from build123d import *

# Parameters (mm, degrees)
F1_DEPTH    = 2.54
F2_T1_DEPTH = 76.5641495789
F3_R        = 2.54
F4_DEPTH    = 2.54


# Not quite as in the source:
# - a fillet or chamfer that OpenCascade refuses, or shapes differently, is made with other operations: its cross-section is extruded or revolved along the edge and cut away or added


with BuildPart() as f1:
    # F0 (on Front) → F1 (new body)
    with BuildSketch(Plane.XZ):
        with BuildLine():
            Line((-63.5, 0), (0, 0))
            Line((0, 0), (-12.7, 19.05))
            Line((-12.7, 19.05), (-19.05, 19.05))
            Line((-19.05, 19.05), (-19.05, 13.97))
            ThreePointArc((-19.05, 13.97), (-22.225, 10.795), (-25.4, 13.97))
            Line((-25.4, 13.97), (-25.4, 19.05))
            Line((-25.4, 19.05), (-38.1, 19.05))
            Line((-38.1, 19.05), (-38.1, 13.97))
            ThreePointArc((-38.1, 13.97), (-41.275, 10.795), (-44.45, 13.97))
            Line((-44.45, 13.97), (-44.45, 19.05))
            Line((-44.45, 19.05), (-50.8, 19.05))
            Line((-50.8, 19.05), (-63.5, 0))
        make_face()
    extrude(amount=F1_DEPTH)

    # F2: chamfer of 2.54 on 2 edges, made by hand

    # F2_s2 → F2_t1 (cut)
    with BuildSketch(Plane.YZ.offset(-70.0320747894)):
        Polygon((0, 0), (-2.54, 2.54), (-2.54, 0), align=None)
        Polygon((-2.54, 0), (0, 2.54), (0, 0), align=None)
    extrude(amount=F2_T1_DEPTH, mode=Mode.SUBTRACT)

    # F3 (on face) → F4 (cut)
    with BuildSketch(Plane.XZ.offset(2.54)):
        with Locations((-12.7, 7.62)):
            Circle(F3_R)
        with Locations((-49.9533333333, 7.62)):
            Circle(F3_R)
    extrude(amount=-F4_DEPTH, mode=Mode.SUBTRACT)


solid = f1.part
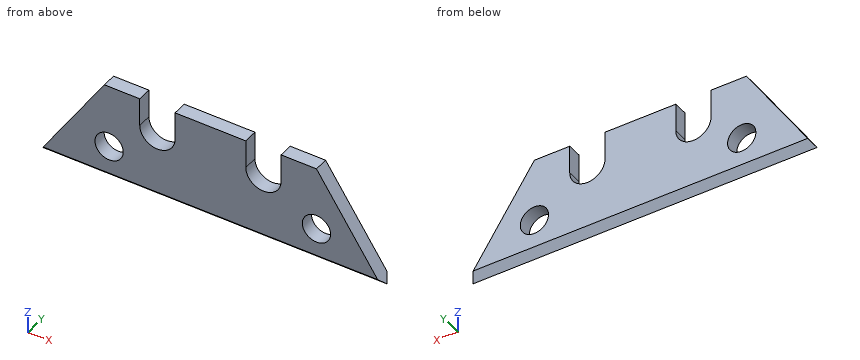
Model file for the job. Use its own axes, mm. Give positions to 0.01 mm unless a question says otherwise; leave off trailing zeros. Loops run counter-clockwise (first coordinate to the right, second up) from the corner with the lowest first, then second, coordinate; pieces in that order, holes last.
Item 1: Drop flat-ended pins along their axis: P1, Ø1.5, axis at y = -0.5, z = 11.5, coming from the -X side; P2, Ø0.8, axis at y = -2, z = 17.5, coming from the +X side; P3, Ø1.3, axis at y = -1.5, z = 16.5, coming from the -X side; P4, Ø4, axis at x = -49.95, z = 7.62, coming from the +Y side. Give the stop position or say it passes through.
Check values:
P1: stops at x = -56.33
P2: stops at x = -11.4
P3: stops at x = -52.93
P4: passes through
Item 2: Slice it at D-D (z = 12). Write the cut outline in (x, y).
Check values:
outline: (-55.5, -2.54) - (-43.76, -2.54) - (-43.76, 0) - (-55.5, 0) - close; (-38.79, -2.54) - (-24.71, -2.54) - (-24.71, 0) - (-38.79, 0) - close; (-19.74, -2.54) - (-8, -2.54) - (-8, 0) - (-19.74, 0) - close
Item 3: Slice it at C-C (x = -49). Write the cut outline in (y, z), plus the area to 3 significant figures.
Check values:
outline: (-2.54, 2.54) - (-1.27, 1.27) - (0, 2.54) - (0, 5.27) - (-2.54, 5.27) - close; (-2.54, 9.97) - (0, 9.97) - (0, 19.05) - (-2.54, 19.05) - close
area: 31.6 mm2
Item 4: Drill centre lines: line 1 along X through (y, z) = (-2.1, 16.5); line 2 along X through (y, z) = (-1.35, 14.25); line 3 along Z through (x, y) = (-12, -0.9). Where is each one in solid material? Low to high.
Check values:
line 1: x = -52.5 to -44.45, -38.1 to -25.4, -19.05 to -11
line 2: x = -54 to -44.45, -38.1 to -25.4, -19.05 to -9.5
line 3: z = 1.64 to 5.18, 10.06 to 18
Item 5: Slice it at A-A (z = 7.62). Write the cut outline in (x, y).
Check values:
outline: (-58.42, -2.54) - (-52.49, -2.54) - (-52.49, 0) - (-58.42, 0) - close; (-47.41, -2.54) - (-15.24, -2.54) - (-15.24, 0) - (-47.41, 0) - close; (-10.16, -2.54) - (-5.08, -2.54) - (-5.08, 0) - (-10.16, 0) - close
Item 6: Slice it at B-B (y = -0.7). Write the cut outline in (x, z) (3 decimals), plus the area to 3 significant figures.
Check values:
outline: (-62.273, 1.84) - (-1.227, 1.84) - (-12.7, 19.05) - (-19.05, 19.05) - (-19.05, 13.97) arc R3.175 cw to (-25.4, 13.97) - (-25.4, 19.05) - (-38.1, 19.05) - (-38.1, 13.97) arc R3.175 cw to (-44.45, 13.97) - (-44.45, 19.05) - (-50.8, 19.05) - close; hole circle Ø5.08 at (-49.953, 7.62); hole circle Ø5.08 at (-12.7, 7.62)
area: 716 mm2
